Drawing for the job (mm, zero at the part's lowest x, y, z). A direction names the side the tool comes from. Coordinates: 2 decimals unless noted, no trailing zeros. Order: outer loops, then holes, each group sorted by start corner. A loop starts at its lowest first (then second) coordinate and runs counter-clockwise, first axis right, second up. Notation, with made-up numbers: M 44.5,64 L 56.5,64 A21 cw 56.5,82 Z; hole C 33.25,-10 d11. An arc over 180 degrees is marked long. Write item = value, one per line. Start each with the question number.
Q1. Pull direction X, two halves, no side cores. Call the marked faces 4, 5 and 6: released by +X, released by -X, zero draft, split by the parting line, or undercut.
Q2. Band-saw the part on D-D on y = 3. Write the cut outline in (x, z).
Q3. Band-saw the part on C-C on x = 4.1. Write the cut outline in (y, z).
Q4. Pin check, flat tips, straight feed: P1, Ø2, axis at x = 0.5, y = 1, coming from the +Z side; P2, Ø0.8, axis at x = 3, z = 2.5, coming from the +Y side. Stop position of each tip, or through.
Q5. Band-saw the part on B-B on z = 2.7. Write the cut outline in (x, y).
Q6. Band-saw the part on A-A on y = 8. Write the cut outline in (x, z).
Q7. Drill centre lines: probe 1 along Y at (x, z) = (3.4, 2.5); probe 2 along Y at (x, z) = (2.65, 0.95); probe 3 along X at (y, z) = (7.75, 1.5). Where is each one in solid material? Low to high.
Q8. 3-axis set-ups, long thin cutter, end or side, ignore diameter. For the marked faces 1, 2 and 3: which of +Z, -Z, +X, -X, +Y, -Y reach the whole face in a straight line?
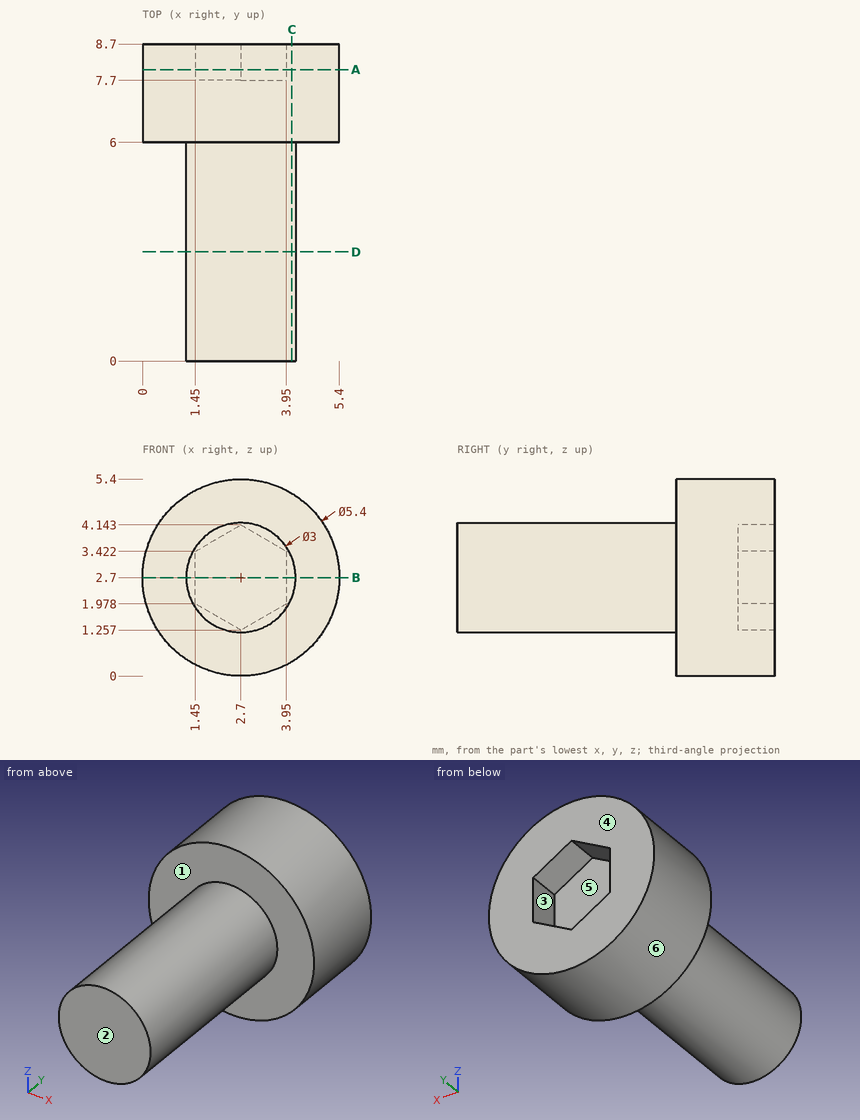
Recorded:
q1.face_4 = zero draft
q1.face_5 = undercut
q1.face_6 = split by the parting line
q2.outline = C 2.7,2.7 d3
q3.outline = M 0,2.16 L 6,2.16 L 6,0.39 L 8.7,0.39 L 8.7,5.01 L 6,5.01 L 6,3.24 L 0,3.24 Z
q4.P1 = 3.6
q4.P2 = 7.7
q5.outline = M 0,6 L 1.2,6 L 1.2,0 L 4.2,0 L 4.2,6 L 5.4,6 L 5.4,8.7 L 3.95,8.7 L 3.95,7.7 L 1.45,7.7 L 1.45,8.7 L 0,8.7 Z
q6.outline = C 2.7,2.7 d5.4; hole M 1.45,1.98 L 2.7,1.26 L 3.95,1.98 L 3.95,3.42 L 2.7,4.14 L 1.45,3.42 Z
q7.probe_1 = 0 to 7.7
q7.probe_2 = 6 to 8.7
q7.probe_3 = 0.28 to 2.28, 3.12 to 5.12
q8.face_1 = -Y
q8.face_2 = +Z, -Z, +X, -X, -Y
q8.face_3 = +Y
